For this review, take the finished solid that the model builds, in its own axes (mm). Coordinates: 2 decimals unless noted, no trailing zeros. Order: outer loops, then holes, each group sorted by start corner. A loop starts at its lowest first (then second) coordinate and runs counter-clockwise, first axis right, second up. Notation, with made-up numbers: (84.5, 13.25) - (124.5, 13.25) arc R32 ccw to (124.5, 42.25) - close; hole circle Ø7 at (-0.75, 54.25). An arc over 180 degrees is marked (long way). One line per item, written item: value. Start each with the question number.
(1) Clearance check with flat-ended pins moving along their axes: pin 1 (8 mm diameter, centred on x = 6.5, y = -174, fed in from +Z); pin 2 (10 mm diameter, centred on x = 4.5, z = 155.5, fed in from +Y); pin 3 (10 mm diameter, centred on y = 176.78, z = -176.78, fed in from +X); pin 4 (2 mm diameter, centred on x = 6.5, y = -106.5, fed in from -Z). State where each tip first meets the part, or that it passes through.
(2) Mouldability with a two-part tool opening along Y and no side actions: class faces 1 (the cylindrical face through (10.14, 180.641, -181.816)), 2 (the cylindrical face through (9.86, 78.097, -247.994)), 3 (the flat face through (20, 4, 4)) as released by +Y, released by -Y, zero draft, split by the parting line, or undercut.
(3) To check wall thickness, follow line 1 along Y through (x, z) = (8.5, 0); line 2 along Z through (x, y) = (10, -0.5); line 3 along Y through (x, z) = (2, -172). State the ranges of each line that lie inside material, in increasing order.
(4) Consider section A-A on z = 0. Write out the cut boundary in (x, y), then the cut area to 3 significant figures.
(5) Consider section C-C on y = -250. Write out the cut boundary in (x, z), then the cut area to 3 significant figures.
(6) Consider section D-D on z = -149. Write out the cut boundary in (x, y), then the cut area to 3 significant figures.
(7) Consider section B-B on x = 11.25. Write out the cut boundary in (y, z), then the cut area to 3 significant figures.
```python
from build123d import *

# Parameters (mm, degrees)
SKETCH1_R                         = 260
BOSS_EXTRUDE1_DEPTH               = 20
F_1_2_13_TAPPED_HOLE1_D           = 10.71626
F_1_2_13_TAPPED_HOLE1_DEPTH       = 70.4
F_1_2_13_TAPPED_HOLE1_CBORE_D     = 12.7
F_1_2_13_TAPPED_HOLE1_CBORE_DEPTH = 64.5
F_1_2_13_TAPPED_HOLE1_TIP         = 3.219489309


with BuildPart() as part:
    # Sketch1 → Boss-Extrude1 (new body)
    with BuildSketch(Plane(origin=(0, 0, 0), x_dir=(0, 0, -1), z_dir=(1, 0, 0))):
        Circle(SKETCH1_R)
    extrude(amount=BOSS_EXTRUDE1_DEPTH)

    # 1/2-13 Tapped Hole1
    with Locations(Plane(origin=(20, 176.776695297, 176.776695297), x_dir=(0, 0, 1), z_dir=(1, 0, 0))):
        with Locations((0, 0), (-353.553390594, 0), (-176.776695297, 426.776695297), (-176.776695297, 325.879201874)):
            CounterBoreHole(F_1_2_13_TAPPED_HOLE1_D / 2, F_1_2_13_TAPPED_HOLE1_CBORE_D / 2, F_1_2_13_TAPPED_HOLE1_CBORE_DEPTH, depth=F_1_2_13_TAPPED_HOLE1_DEPTH)
            with Locations((0, 0, -(F_1_2_13_TAPPED_HOLE1_DEPTH + F_1_2_13_TAPPED_HOLE1_TIP / 2))):  # 118° drill point
                Cone(0, F_1_2_13_TAPPED_HOLE1_D / 2, F_1_2_13_TAPPED_HOLE1_TIP, mode=Mode.SUBTRACT)


solid = part.part
```
Geometry check:
1. pin 1: stops at z = 196.72
1. pin 2: stops at y = 212.01
1. pin 3: passes through
1. pin 4: stops at z = -237.63
2. face 1: undercut
2. face 2: split by the parting line
2. face 3: zero draft
3. line 1: y = -260 to -256.35, -243.65 to -155.45, -142.75 to 260
3. line 2: z = -260 to 260
3. line 3: y = -194.98 to 172.59, 180.96 to 194.98
4. outline: (0, -260) - (20, -260) - (20, -256.35) - (0, -256.35) - close; (0, -243.65) - (20, -243.65) - (20, -155.45) - (0, -155.45) - close; (0, -142.75) - (20, -142.75) - (20, 260) - (0, 260) - close
4. area: 9,890 mm^2
5. outline: (0, -71.41) - (20, -71.41) - (20, -6.35) - (0, -6.35) - close; (0, 6.35) - (20, 6.35) - (20, 71.41) - (0, 71.41) - close
5. area: 2,600 mm^2
6. outline: (0, -213.07) - (20, -213.07) - (20, 213.07) - (0, 213.07) - close
6. area: 8,520 mm^2
7. outline: circle Ø520 at (0, 0); hole circle Ø12.7 at (-250, 0); hole circle Ø12.7 at (-149.1, 0); hole circle Ø12.7 at (176.78, -176.78); hole circle Ø12.7 at (176.78, 176.78)
7. area: 212,000 mm^2
